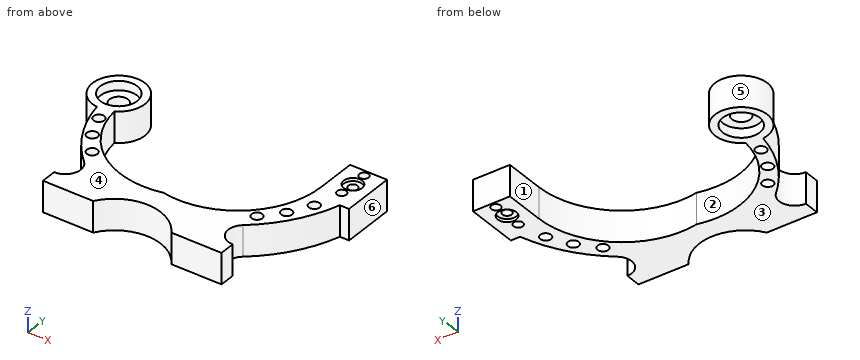
```python
from build123d import *

# Parameters (mm, degrees)
EXTRUDE_1_DEPTH          = 5
SKETCH_2_R               = 3
CUT_EXTRUDE_1_DEPTH      = 1
CUT_EXTRUDE_2_DEPTH      = 91.056926441
CUT_EXTRUDE_2_DEPTH_BACK = 91.056926441
SKETCH_3_R               = 1.5
SKETCH_4_R               = 1.5
CUT_EXTRUDE_3_DEPTH      = 91.162353563
SKETCH_5_R               = 1.75
CUT_EXTRUDE_4_DEPTH      = 91.162353563
CUT_EXTRUDE_START        = -3
SKETCH_6_R               = 6
CUT_EXTRUDE_5_DEPTH      = 94.162353563
SKETCH_7_R               = 3
CUT_EXTRUDE_6_DEPTH      = 90.879085443


with BuildPart() as part:
    # Sketch 1 → Extrude 1 (new, symmetric)
    with BuildSketch(Plane(origin=(0, 0, 0), x_dir=(-1, 0, 0), z_dir=(0, 0, -1))):
        with BuildLine():
            Line((-7.5, 6), (8.81142246, 6))
            ThreePointArc((8.81142246, 6), (21.5, 13), (34.18857754, 6))
            Line((34.18857754, 6), (50.5, 6))
            Line((50.5, 6), (50.5, 11))
            ThreePointArc((50.5, 11), (45.852558058, 14.155743132), (47.071569313, 19.639486643))
            ThreePointArc((47.071569313, 19.639486643), (55.125553128, 30.1016183), (59.5, 42.559028492))
            ThreePointArc((59.5, 42.559028492), (60.072054975, 59.353361189), (54.5, 43.5))
            ThreePointArc((54.5, 43.5), (43.306585473, 24.298199123), (21.5, 20))
            ThreePointArc((21.5, 20), (-0.73368794, 25.748388632), (-10.5, 46.532998323))
            Line((-10.5, 46.532998323), (-10.5, 59.5))
            Line((-10.5, 59.5), (-22.5, 59.5))
            Line((-22.5, 59.5), (-22.5, 42.5))
            Line((-22.5, 42.5), (-19.5, 42.5))
            ThreePointArc((-19.5, 42.5), (-13.686520363, 30.033883058), (-4.37890781, 19.906249293))
            ThreePointArc((-4.37890781, 19.906249293), (-2.781353665, 14.346404897), (-7.5, 11))
            Line((-7.5, 11), (-7.5, 6))
        make_face()
    extrude(amount=EXTRUDE_1_DEPTH, both=True)

    # Sketch 2 → Cut-Extrude 1 (cut)
    with BuildSketch(Plane.XY.offset(5)):
        with Locations((16.5, 52.5)):
            Circle(SKETCH_2_R)
    cut_extrude_1 = extrude(amount=-CUT_EXTRUDE_1_DEPTH, mode=Mode.SUBTRACT)

    # Sketch 3 → Cut-Extrude 2 (cut, two sides: drawn at the far end of the back side and taken through both)
    with BuildSketch(Plane.XY.offset(4).offset(-CUT_EXTRUDE_2_DEPTH_BACK)):
        with Locations((16.5, 52.5)):
            Circle(SKETCH_3_R)
    extrude(amount=CUT_EXTRUDE_2_DEPTH + CUT_EXTRUDE_2_DEPTH_BACK, mode=Mode.SUBTRACT)

    # Sketch 4 → Cut-Extrude 3 (cut, through all)
    with BuildSketch(Plane.XY.offset(5)):
        with Locations((16.5, 57.5)):
            Circle(SKETCH_4_R)
        with Locations((16.5, 47.5)):
            Circle(SKETCH_4_R)
    extrude(amount=-CUT_EXTRUDE_3_DEPTH, mode=Mode.SUBTRACT)

    # Sketch 5 → Cut-Extrude 4 (cut, through all)
    with BuildSketch(Plane.XY.offset(5)):
        with Locations((14.099159256, 38.5)):
            Circle(SKETCH_5_R)
        with Locations((10.191784732, 31.519138712)):
            Circle(SKETCH_5_R)
        with Locations((4.897441914, 25.521644724)):
            Circle(SKETCH_5_R)
        with Locations((-55.897925178, 38.5)):
            Circle(SKETCH_5_R)
        with Locations((-52.723592313, 31.156730234)):
            Circle(SKETCH_5_R)
        with Locations((-48.053046301, 24.661655181)):
            Circle(SKETCH_5_R)
    extrude(amount=-CUT_EXTRUDE_4_DEPTH, mode=Mode.SUBTRACT)

    # Mirror 1: Cut-Extrude 1 across plane
    add(cut_extrude_1.mirror(Plane(origin=(0, 0, 0), x_dir=(1, 0, 0), z_dir=(0, 0, -1))), mode=Mode.SUBTRACT)

    # Sketch 6 → Cut-Extrude 5 (cut)
    with BuildSketch(Plane.XY.offset(5).offset(CUT_EXTRUDE_START)):
        with Locations(Location((-58.5, 51, 0), (0, 0, 180))):
            Circle(SKETCH_6_R)
    cut_extrude_5 = extrude(amount=CUT_EXTRUDE_5_DEPTH, mode=Mode.SUBTRACT)

    # Mirror 2: Cut-Extrude 5 across plane
    add(cut_extrude_5.mirror(Plane.XY), mode=Mode.SUBTRACT)

    # Sketch 7 → Cut-Extrude 6 (cut, through all)
    with BuildSketch(Plane.XY.offset(2)):
        with Locations((-58.5, 51)):
            Circle(SKETCH_7_R)
    extrude(amount=-CUT_EXTRUDE_6_DEPTH, mode=Mode.SUBTRACT)


solid = part.part
```
Can you work these out from the model? Positions are in its coordinate system, mm. Face numbers are marked on the shaded views. A direction names the side the tool comes from. Give positions to 0.01 mm unless a question says otherwise; leave off trailing zeros. Write each loop counter-clockwise with the first axis right and the second up, starting at its lowest first coordinate (ties: lowest second). Pieces come first, ordered by that corner, then holes. Notation, with made-up numbers: (58.5, 54.25) - (72.5, 54.25) arc R29 ccw to (72.5, 75.25) - close; hole circle Ø10 at (1, 49.25). An arc over 180 degrees is marked (long way). Write item = value, one per line. Start each with the question number.
1. Imagine slicing it at D-D (y = 21.5). Please give me the cut outline in (x, z).
2. On a 3-axis mill with a long thin cutter (end or side, diameter ignored), from which of +Z, -Z, +X, -X, +Y, -Y can I reach the whole of each face in a straight line? I mean the marked faces 1, 2 and 3. Say none if no direction works.
3. Imagine slicing it at A-A (x = -58.5). Please give me the cut outline in (y, z).
4. Imagine slicing it at B-B (y = 52.5). Count the separate pieces of the cut face and the enclosed holes in it, and give its area (3 significant figures).
5. Please list where these lines run through material, in increasing order: line 1 (Y direction, x = 16.5, z = -4.45); line 2 (Y direction, x = -49.5, z = -3.25); line 3 (X direction, y = 32, z = 1.5).
6. For pin 1 (1.5 mm diameter, centred on y = 46.5, z = -3.5, fed in from -X); pin 2 (1.5 mm diameter, centred on y = 9.5, z = 0.5, fed in from +X); pin 3 (2.5 mm diameter, centred on x = 21.5, z = 1, fed in from -Y); pin 4 (3.5 mm diameter, centred on x = -58.5, y = 51, fed in from -Z), each with a flat end and sliding along its axis, tell me the tip position at first contact or that it passes through.
7. Thinking about a two-plate mould opening in X: for the marked faces 4, 5 and 6, which applies, released by +X, released by -X, zero draft, split by the parting line, or undercut?
Worked answers:
q1.outline = (-48.93, -5) - (-38.34, -5) - (-38.34, 5) - (-48.93, 5) - close; (-6.38, -5) - (6.27, -5) - (6.27, 5) - (-6.38, 5) - close
q2.face_1 = +Z, -Z, +Y
q2.face_2 = +Z, -Z
q2.face_3 = -Z, +X, -X, +Y, -Y
q3.outline = (38.31, -5) - (45, -5) - (45, -2) - (48, -2) - (48, 2) - (45, 2) - (45, 5) - (38.31, 5) - close; (54, -2) - (57, -2) - (57, -5) - (59.5, -5) - (59.5, 5) - (57, 5) - (57, 2) - (54, 2) - close
q4.separate_pieces = 4
q4.enclosed_holes = 0
q4.area = 161 mm2
q5.line_1 = 34.86 to 46, 49 to 49.5, 55.5 to 56, 59 to 59.5
q5.line_2 = 6 to 11.1, 22.13 to 23.68, 25.65 to 30.44
q5.line_3 = -56.09 to -54.26, -51.19 to -50.55, 6.26 to 8.51, 11.87 to 14.93
q6.pin_1 = -66.13
q6.pin_2 = 7.5
q6.pin_3 = 42.5
q6.pin_4 = through
q7.face_4 = zero draft
q7.face_5 = undercut
q7.face_6 = released by +X
